from build123d import *

# Parameters (mm, degrees)
BOSS_EXTRUDE1_DEPTH     = 161.208217
BOSS_EXTRUDE2_DEPTH     = 4
BOSS_EXTRUDE3_DEPTH     = 10
BOSS_EXTRUDE4_DEPTH     = 4
SKETCH6_R               = 2
CUT_EXTRUDE1_DEPTH      = 74.097308941
CUT_EXTRUDE1_DEPTH_BACK = 66.896441548


with BuildPart() as part:
    # Sketch1 → Boss-Extrude1 (new body)
    with BuildSketch(Plane.XY):
        with BuildLine():
            Line((50, 64.298335316), (48, 64.298335316))
            ThreePointArc((48, 64.298335316), (0, 16.298335316), (-48, 64.298335316))
            Line((-48, 64.298335316), (-50, 64.298335316))
            ThreePointArc((-50, 64.298335316), (0, 14.298335316), (50, 64.298335316))
        make_face()
    extrude(amount=BOSS_EXTRUDE1_DEPTH)

    # Sketch3 → Boss-Extrude2 (add)
    with BuildSketch(Plane.XY.offset(161.208216537)):
        with BuildLine():
            Line((50, 64.298335316), (48, 64.298335316))
            ThreePointArc((48, 64.298335316), (0, 16.298335316), (-48, 64.298335316))
            Line((-48, 64.298335316), (-50, 64.298335316))
            ThreePointArc((-50, 64.298335316), (0, 14.298335316), (50, 64.298335316))
        make_face()
    extrude(amount=BOSS_EXTRUDE2_DEPTH)



with BuildPart() as body_2:
    # Sketch4 → Boss-Extrude3 (new body)
    with BuildSketch(Plane.XY.offset(165.208216537)):
        with BuildLine():
            Line((-54, 64.298335316), (-52, 64.298335316))
            ThreePointArc((-52, 64.298335316), (0, 12.298335316), (52, 64.298335316))
            Line((52, 64.298335316), (54, 64.298335316))
            ThreePointArc((54, 64.298335316), (0, 10.298335316), (-54, 64.298335316))
        make_face()
    extrude(amount=-BOSS_EXTRUDE3_DEPTH)


with BuildPart() as part_1:
    add(part.part)

    add(body_2.part)  # Boss-Extrude4 merges body 2
    # Sketch5 → Boss-Extrude4 (add)
    with BuildSketch(Plane.XY.offset(165.208216537)):
        with BuildLine():
            Line((-50, 64.298335316), (-52, 64.298335316))
            ThreePointArc((-52, 64.298335316), (0, 12.298335316), (52, 64.298335316))
            Line((52, 64.298335316), (50, 64.298335316))
            ThreePointArc((50, 64.298335316), (0, 14.298335316), (-50, 64.298335316))
        make_face()
    extrude(amount=-BOSS_EXTRUDE4_DEPTH)

    # Sketch6 → Cut-Extrude1 (cut, two sides)
    with BuildSketch(Plane(origin=(0, 66.78809677, 46.765528821), x_dir=(-1, 0, 0), z_dir=(0, -0.819152044, -0.573576436))) as cut_extrude1_sk:
        with Locations((-8, -80)):
            Circle(SKETCH6_R)
        with Locations((8, -80)):
            Circle(SKETCH6_R)
        with Locations((8, -45)):
            Circle(SKETCH6_R)
        with Locations((-8, -45)):
            Circle(SKETCH6_R)
        with BuildLine():
            Line((-15, -128.204829529), (-15, -45))
            ThreePointArc((-15, -45), (-12.949747468, -40.050252532), (-8, -38))
            Line((-8, -38), (8, -38))
            ThreePointArc((8, -38), (12.949747468, -40.050252532), (15, -45))
            Line((15, -45), (15, -128.204829529))
            add(Edge.make_bspline(
                [(15, -128.204829529), (54, -121.736527083), (54, -98.450638275)],
                knots=[1.8522764, 1.8522764, 1.8522764, 3.141592654, 3.141592654, 3.141592654], degree=2, weights=[1, 0.799305254, 1]))
            Line((54, -98.450638275), (54, 36.880010034))
            Line((54, 36.880010034), (-54, 36.880010034))
            Line((-54, 36.880010034), (-54, -98.450638275))
            add(Edge.make_bspline(
                [(-54, -98.450638275), (-54, -121.736527083), (-15, -128.204829529)],
                knots=[0, 0, 0, 1.289316254, 1.289316254, 1.289316254], degree=2, weights=[1, 0.799305254, 1]))
        make_face()
    extrude(amount=CUT_EXTRUDE1_DEPTH, mode=Mode.SUBTRACT)
    extrude(cut_extrude1_sk.sketch, amount=-CUT_EXTRUDE1_DEPTH_BACK, mode=Mode.SUBTRACT)


solid = part_1.part
The model under review builds one solid part; all positions refer to its coordinate system, in mm. A direction names the side the tool comes from. Coordinates: 2 decimals unless noted, no trailing zeros. Write each loop counter-clockwise with the first axis right and the second up, starting at its lowest first coordinate (ties: lowest second). Pieces come first, ordered by that corner, then holes. Notation, with made-up numbers: M 38,4 L 84,4 A20 ccw 84,11 Z; hole C 52.5,49.5 d1. An arc over 180 degrees is marked long. Put each result on its own line as item: value.
1) Wall thickness on probe 1 along Z at (x, y) = (1, 13); probe 2 along Z at (x, y) = (9, 12.25); probe 3 along Y at (x, z) = (1, 129): over which ranges is each line inside the solid? List them lowest first. Write a range as [from, to].
Computed:
probe 1: z = [161.21, 165.21]
probe 2: z = [155.21, 165.21]
probe 3: y = [14.31, 16.31]
2) For faces 5 (the cylindrical face through (-0.2, 12.3, 158.3)), 6 (the cylindrical face through (-12.93, 17.11, 60.85)), list the 3-axis set-ups (+Z, -Z, +X, -X, +Y, -Y) from which the entire face can be reached by the end or side of a thin tool; tool diameter is ignored.
Computed:
face 5: -Z
face 6: -Z, -X, +Y
3) Add section B-B on x = -0.5. Give the boundary of the cut face in (y, z).
Computed:
outline: M 10.3,155.21 L 12.3,155.21 L 12.3,161.21 L 14.3,161.21 L 14.3,56.4 L 16.3,57.8 L 16.3,165.21 L 10.3,165.21 Z
4) Add section C-C on z = 85. Give the boundary of the cut face in (x, y).
Computed:
outline: M -15,16.6 A50 ccw 15,16.6 L 15,18.7 A48 cw -15,18.7 Z
5) Add section D-D on x = -5. Give the boundary of the cut face in (y, z).
Computed:
outline: M 10.53,155.21 L 12.54,155.21 L 12.54,161.21 L 14.55,161.21 L 14.55,56.58 L 16.56,57.98 L 16.56,165.21 L 10.53,165.21 Z
6) Draft analysis for pull direction Z (two halves, no side actions). For faces 1 (the cylindrical face through (-9.908, 16.337, 108.368)), 2 (the flat face through (0, 14, 165.208)), 3 (the cylindrical face through (10, 16, 66.1)), 4 (the flat face through (0.11, 15.65, 57.35)), state which applies: released by +Z, released by -Z, zero draft, split by the parting line, or undercut.
Computed:
face 1: undercut
face 2: released by +Z
face 3: undercut
face 4: released by -Z
7) Add section A-A on z = 156.5. Give the boundary of the cut face in (x, y), then the cut area to 3 significant figures.
Computed:
outline: M -15,12.42 A54 ccw 15,12.42 L 15,14.51 A52 cw -15,14.51 Z; M -15,16.6 A50 ccw 15,16.6 L 15,18.7 A48 cw -15,18.7 Z
area: 122 mm2
8) Clearance check with flat-ended pins moving along their axes: pin 1 Ø2 at (x, y) = (-3, 12) entering from -Z; pin 2 Ø1.3 at (x, y) = (2.5, 14) entering from -Z; pin 3 Ø12 at (x, z) = (1, 109) entering from -Y. State where each tip first meets the part, or that it passes through.
Computed:
pin 1: stops at z = 155.21
pin 2: stops at z = 56.43
pin 3: stops at y = 14.3
